Here's how the part is built. I have some questions about the finished solid (model axes, mm). Face numbers are marked on the shaded views. A direction names the side the tool comes from. Round coordinates to 2 decimals unless told otherwise and drop trailing zeros. Write each loop counter-clockwise with the first axis right and the second up, starting at its lowest first coordinate (ties: lowest second). Pieces come first, ordered by that corner, then holes. Notation, with made-up numbers: M -19,-31 L 4,-31 A16 ccw 4,-21 Z; hole C -27.5,-1 d9. An arc over 180 degrees is marked long. Write item = value, one per line. Start each with the question number.
(1) I want a section at D-D (x = -5.5). List the corners of the cut face in (y, z) for me, and give its area (3 significant figures).
(2) I want a section at C-C (y = -20). List the corners of the cut face in (x, z) for me.
(3) I need wall thicknesses on line 1 along Z through (x, y) = (-15, -2); line 2 along Y through (x, z) = (-2, 46); line 3 along Z through (x, y) = (1, -16.5). Which ranges of each line are inside material? Lowest first, please.
(4) Will these pins go through, and if not, where does the flat tip stop? pin 1 Ø2.5 at (x, z) = (-15, 47.5) entering from -Y; pin 2 Ø6 at (y, z) = (-13, 23.5) entering from +X; pin 3 Ø2 at (x, y) = (2, -22) entering from +Z; pin 4 Ø4 at (x, z) = (-20.5, 15) entering from -Y.
(5) If we mould it in two halves opening along Z, with no side actions, what happens to the marked faces 3, 4, 5 and 6? For each: released by +Z, released by -Z, zero draft, split by the parting line, or undercut.
(6) I want a section at B-B (x = -15). List the corners of the cut face in (y, z) for me.
(7) On a 3-axis mill with a long thin cutter (end or side, diameter ignored), from which of +Z, -Z, +X, -X, +Y, -Y can I reach the whole of each face in a straight line? I mean the marked faces 1 and 2. Say none if no direction works.
(8) I want a section at A-A (z = 28). List the corners of the cut face in (x, y) for me, and give its area (3 significant figures).
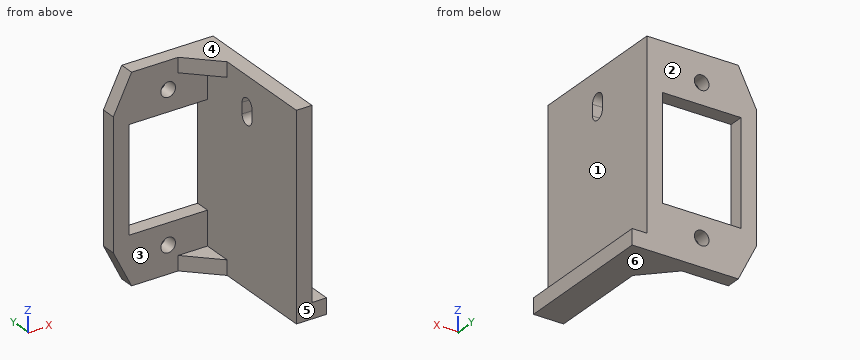
```python
from build123d import *

# Parameters (mm, degrees)
F0_W      = 30
F0_H      = 55
F0_R      = 2
F0_W_2    = 21.5
F0_H_2    = 28.5
F1_DEPTH  = 4
F3_DEPTH  = 36
F5_DEPTH  = 4
F7_W      = 4
F7_H      = 4.25
F8_DEPTH  = 4
F10_DEPTH = 4
F11_DEPTH = 8.251
F12_SIZE2 = 10
F12_SIZE  = 5


with BuildPart() as f1:
    # F0 (on Front) → F1 (new body)
    with BuildSketch(Plane.XZ):
        with Locations((-15, 27.5)):
            Rectangle(F0_W, F0_H)
        with Locations((-15, 7.5)):
            Circle(F0_R, mode=Mode.SUBTRACT)
        with Locations((-15, 27.5)):
            Rectangle(F0_W_2, F0_H_2, mode=Mode.SUBTRACT)
        with Locations((-15, 47.5)):
            Circle(F0_R, mode=Mode.SUBTRACT)
    extrude(amount=F1_DEPTH)

    # F2 (on face) → F3 (join)
    with BuildSketch(Plane.XZ.offset(4)):
        Polygon((0, 4.25), (0, 55), (-4.25, 55), (-4.25, 0), (4, 0), (4, 4.25), align=None)
    extrude(amount=F3_DEPTH)

    # F4 (on face) → F5 (join)
    with BuildSketch(Plane.XY.offset(55)):
        Polygon((-4.25, -12), (-4.25, -4), (-12.25, -4), align=None)
    extrude(amount=-F5_DEPTH)

    # F7 (on face) → F8 (join)
    with BuildSketch(Plane(origin=(0, -4, 0), x_dir=(-1, 0, 0), z_dir=(0, 1, 0))):
        with Locations((-2, 2.125)):
            Rectangle(F7_W, F7_H)
    extrude(amount=F8_DEPTH)

    # F9 (on face) → F10 (join)
    with BuildSketch(Plane(origin=(0, 0, 0), x_dir=(1, 0, 0), z_dir=(0, 0, -1))):
        Polygon((-4.25, 12), (-12.25, 4), (-4.25, 4), align=None)
    extrude(amount=-F10_DEPTH)

    # F6 (on face) → F11 (cut, through all)
    with BuildSketch(Plane(origin=(-4.25, 0, 0), x_dir=(0, -1, 0), z_dir=(-1, 0, 0))):
        with BuildLine():
            ThreePointArc((22, 47.25), (20, 49.25), (18, 47.25))
            Line((18, 47.25), (18, 44.25))
            ThreePointArc((18, 44.25), (20, 42.25), (22, 44.25))
            Line((22, 44.25), (22, 47.25))
        make_face()
    extrude(amount=-F11_DEPTH, mode=Mode.SUBTRACT)

    # F12
    f12_edges = [f1.edges().sort_by_distance(p)[0] for p in [
        (-30, -2, 0),
        (-30, -2, 55),
    ]]
    chamfer(f12_edges, length=F12_SIZE, length2=F12_SIZE2)


solid = f1.part
```
Returned:
q1.outline = M -10.75,0 L 0,0 L 0,13.25 L -4,13.25 L -4,4 L -10.75,4 Z; M -10.75,51 L -4,51 L -4,41.75 L 0,41.75 L 0,55 L -10.75,55 Z
q1.area = 160 mm²
q2.outline = M -4.25,0 L 4,0 L 4,4.25 L 0,4.25 L 0,42.25 L -4.25,42.25 Z; M -4.25,49.25 L 0,49.25 L 0,55 L -4.25,55 Z
q3.line_1 = 0 to 5.5, 9.5 to 13.25, 41.75 to 45.5, 49.5 to 55
q3.line_2 = -40 to -22, -18 to 0
q3.line_3 = 0 to 4.25
q4.pin_1 = through
q4.pin_2 = 0
q4.pin_3 = 4.25
q4.pin_4 = -4
q5.face_3 = undercut
q5.face_4 = released by +Z
q5.face_5 = zero draft
q5.face_6 = released by -Z
q6.outline = M -4,0 L 0,0 L 0,5.5 L -4,5.5 Z; M -4,9.5 L 0,9.5 L 0,13.25 L -4,13.25 Z; M -4,41.75 L 0,41.75 L 0,45.5 L -4,45.5 Z; M -4,49.5 L 0,49.5 L 0,55 L -4,55 Z
q7.face_1 = +Z, +X, +Y, -Y
q7.face_2 = +Z, -Z, +X, -X, +Y
q8.outline = M -30,-4 L -25.75,-4 L -25.75,0 L -30,0 Z; M -4.25,-40 L 0,-40 L 0,0 L -4.25,0 Z
q8.area = 187 mm²
